Could you check a few things on this model? Use its own coordinates, in mm. A direction names the side the tool comes from. Give positions to 0.01 mm unless a question says otherwise; leave off trailing zeros. Order: outer loops, then holes, each group sorted by start corner. A loop starts at its lowest first (then second) coordinate and runs counter-clockwise, first axis right, second up.
(1) Imagine slicing it at A-A, the plane x = 20. Write out the boundary of the cut face in (y, z).
(2) Imagine slicing it at C-C, the plane z = 5.5. Write out the boundary of the cut face in (x, y).
(3) On a 3-axis mill with a long thin cutter (end or side, diameter ignored), from which of +Z, -Z, +X, -X, +Y, -Y can I reach the whole of each face in a straight line? I mean faces 1 (the cylindrical face through (-19.83, -0.17, 7.25)), 2 (the flat face through (-30, 0, 5)). Say none if no direction works.
(4) If I drill on probe 1 along X at (y, z) = (-21.5, 13.5); probe 2 along X at (y, z) = (18, 13); probe 3 along Y at (x, z) = (17.5, 9.5), over which ranges is the centre line in solid material (lowest first)?
(5) Imagine slicing it at B-B, the plane y = -6.5. Write out the boundary of the cut face in (x, z), then the cut area to 3 significant figures.
(6) If we mould it in two halves opening along Y, with no side actions, what happens to faces 3 (the flat face through (-35, 0, 12)), 4 (the flat face through (0, 25, 7)), 5 (the flat face through (0, -25, 7)), 6 (the cylindrical face through (20, -1, 10))? For each: released by +Y, released by -Y, zero draft, split by the parting line, or undercut.
(7) Imagine slicing it at D-D, the plane z = 8.75. Write out the boundary of the cut face in (x, y), then the cut area to 3 significant figures.
from build123d import *

# Parameters (mm, degrees)
ESQUISSE1_W                  = 70
ESQUISSE1_H                  = 50
BOSS_EXTRU_1_DEPTH           = 15
ESQUISSE2_R                  = 4.25
ENL_V_MAT_EXTRU_1_DEPTH      = 63.84902545
ENL_V_MAT_EXTRU_2_DEPTH      = 12.25
ENL_V_MAT_EXTRU_2_DEPTH_BACK = 12.25
ESQUISSE3_R                  = 7.75
ESQUISSE4_R                  = 11
ENL_V_MAT_EXTRU_3_DEPTH      = 3
ESQUISSE5_R                  = 5
ENL_V_MAT_EXTRU_4_DEPTH      = 15
CHANFREIN1_SIZE              = 10


with BuildPart() as part:
    # Esquisse1 → Boss.-Extru.1 (new body)
    with BuildSketch(Plane.XY):
        Rectangle(ESQUISSE1_W, ESQUISSE1_H)
    extrude(amount=BOSS_EXTRU_1_DEPTH)

    # Esquisse2 → Enlèv. mat.-Extru.1 (cut, through all)
    with BuildSketch(Plane(origin=(0, 25, 0), x_dir=(1, 0, 0), z_dir=(0, 1, 0))):
        with Locations((-20, -15)):
            Circle(ESQUISSE2_R)
        with Locations((20, -15)):
            Circle(ESQUISSE2_R)
    extrude(amount=-ENL_V_MAT_EXTRU_1_DEPTH, mode=Mode.SUBTRACT)

    # Esquisse3 → Enlèv. mat.-Extru.2 (cut, two sides: drawn at the far end of the back side and taken through both)
    with BuildSketch(Plane(origin=(0, 0, 0), x_dir=(1, 0, 0), z_dir=(0, 1, 0)).offset(-ENL_V_MAT_EXTRU_2_DEPTH_BACK)):
        with Locations((-20, -15)):
            Circle(ESQUISSE3_R)
    extrude(amount=ENL_V_MAT_EXTRU_2_DEPTH + ENL_V_MAT_EXTRU_2_DEPTH_BACK, mode=Mode.SUBTRACT)

    # Esquisse4 → Enlèv. mat.-Extru.3 (cut)
    with BuildSketch(Plane(origin=(0, 7.5, 0), x_dir=(1, 0, 0), z_dir=(0, 1, 0))):
        with Locations((20, -15)):
            Circle(ESQUISSE4_R)
    extrude(amount=-ENL_V_MAT_EXTRU_3_DEPTH, mode=Mode.SUBTRACT)

    # Esquisse5 → Enlèv. mat.-Extru.4 (cut)
    with BuildSketch(Plane(origin=(0, 7.5, 0), x_dir=(1, 0, 0), z_dir=(0, 1, 0))):
        with Locations((20, -15)):
            Circle(ESQUISSE5_R)
    extrude(amount=-ENL_V_MAT_EXTRU_4_DEPTH, mode=Mode.SUBTRACT)

    # Chanfrein1
    chanfrein1_edges = [part.edges().sort_by_distance(p)[0] for p in [
        (-35, 0, 0),
        (35, 0, 0),
    ]]
    chamfer(chanfrein1_edges, length=CHANFREIN1_SIZE)


solid = part.part
Answer block:
1. outline: (-25, 0) - (25, 0) - (25, 10.75) - (7.5, 10.75) - (7.5, 4) - (4.5, 4) - (4.5, 10) - (-7.5, 10) - (-7.5, 10.75) - (-25, 10.75) - close
2. outline: (-30.5, -25) - (30.5, -25) - (30.5, 25) - (-30.5, 25) - close; hole (14.45, 4.5) - (25.55, 4.5) - (25.55, 7.5) - (14.45, 7.5) - close
3. face 1: +Z
3. face 2: -Z, -X, +Y, -Y
4. probe 1: x = -35 to -23.98, -16.02 to 16.02, 23.98 to 35
4. probe 2: x = -35 to -23.75, -16.25 to 16.25, 23.75 to 35
4. probe 3: y = -25 to 4.5, 7.5 to 25
5. outline: (-35, 10) - (-25, 0) - (25, 0) - (35, 10) - (35, 15) - (25, 15) arc R5 cw to (15, 15) - (-12.25, 15) arc R7.75 cw to (-27.75, 15) - (-35, 15) - close
5. area: 816 mm2
6. face 3: zero draft
6. face 4: released by +Y
6. face 5: released by -Y
6. face 6: undercut
7. outline: (-33.75, -25) - (33.75, -25) - (33.75, 25) - (-33.75, 25) - close; hole (-24.58, -12.25) - (-15.42, -12.25) - (-15.42, 12.25) - (-24.58, 12.25) - close; hole (10.95, 4.5) - (29.05, 4.5) - (29.05, 7.5) - (10.95, 7.5) - close
7. area: 3,100 mm2
